Job drawing, mm, ordinate dimensions from the low corner. One solid piece. Round coordinates to 2 decimals unless told otherwise and drop trailing zeros. Write each loop counter-clockwise with the first axis right and the second up, starting at its lowest first coordinate (ties: lowest second). Pieces come first, ordered by that corner, then holes. Notation, with made-up numbers: (-2, -6) - (40, -6) arc R20 cw to (40, 0) - close; hole circle Ø4 at (38, -32.75). An arc over 180 degrees is marked (long way). Write each question's results on one line, items separated by ' | '.
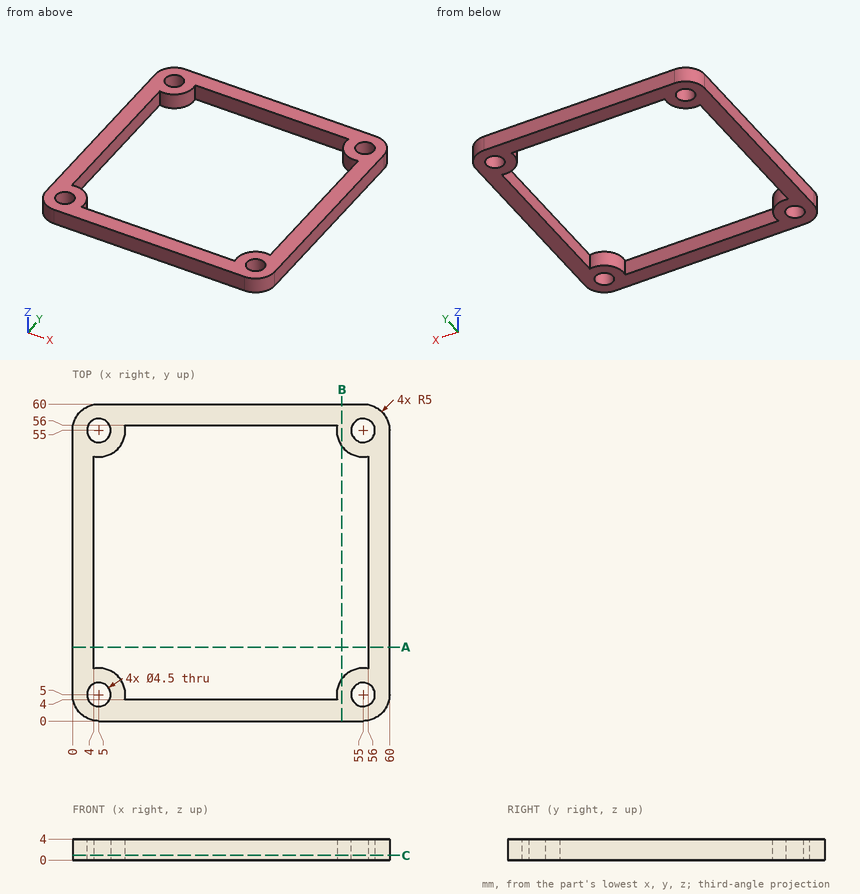
(1) Slice it at C-C, the plane z = 0.9. Write the cut outline in (x, y), and give its area (3 significant figures).
Worked answers:
outline: (0, 5) arc R5 ccw to (5, 0) - (55, 0) arc R5 ccw to (60, 5) - (60, 55) arc R5 ccw to (55, 60) - (5, 60) arc R5 ccw to (0, 55) - close; hole circle Ø4.5 at (5, 5); hole circle Ø4.5 at (5, 55); hole (4, 9.9) arc R5 cw to (9.9, 4) - (50.1, 4) arc R5 cw to (56, 9.9) - (56, 50.1) arc R5 cw to (50.1, 56) - (9.9, 56) arc R5 cw to (4, 50.1) - close; hole circle Ø4.5 at (55, 5); hole circle Ø4.5 at (55, 55) | area: 933 mm2
(2) Drill centre lines: probe 1 along Y at (x, z) = (5, 1.65); probe 2 along X at (y, z) = (22, 3.1). Where is each one in solid material? Low to high. Write a range as [from, to].
Worked answers:
probe 1: y = [0, 2.75], [7.25, 10], [50, 52.75], [57.25, 60] | probe 2: x = [0, 4], [56, 60]
(3) Slice it at A-A, the plane y = 14. Write the cut outline in (x, z).
Worked answers:
outline: (0, 0) - (4, 0) - (4, 4) - (0, 4) - close; (56, 0) - (60, 0) - (60, 4) - (56, 4) - close
(4) Slice it at B-B, the plane x = 51. Write the cut outline in (y, z), and give its area (3 significant figures).
Worked answers:
outline: (0, 0) - (8, 0) - (8, 4) - (0, 4) - close; (52, 0) - (60, 0) - (60, 4) - (52, 4) - close | area: 64.0 mm2
